Input: part model. Units: mm. Frame: model coordinates. A direction names the side the tool comes from. Give positions to 0.01 mm unless a question says otherwise; leave off trailing zeros. Write each loop counter-clockwise with the first axis right and the second up, starting at its lowest first coordinate (ties: lowest second). Pieces come first, ordered by that corner, then holes. Notation, with made-up numbers: (68, 18.5) - (73, 18.5) arc R6 ccw to (73, 26.5) - close; hole circle Ø7 at (40.5, -39.75). An arc over 180 degrees is marked (long way). Answer as a JSON object with one key per item and string values. Group by question number.
Autodesk Inventor part; units mm, degrees
ref_plane "YZ Plane" through (0, 0, 0) normal (1, 0, 0) x (0, 1, 0)
ref_plane "XZ Plane" through (0, 0, 0) normal (0, 1, 0) x (-1, 0, 0)
ref_plane "XY Plane" through (0, 0, 0) normal (0, 0, 1) x (1, 0, 0)
sketch "Boceto1" plane through (0, 0, 0) normal (0, 0, 1) x (1, 0, 0)
  line L0 (-225.8925, 111.7519) -> (-185.8925, 111.7519)
  line L1 (-185.8925, 111.7519) -> (-185.8925, 71.7519)
  line L2 (-225.8925, 101.7519) -> (-195.8925, 101.7519)
  line L3 (-195.8925, 101.7519) -> (-195.8925, 71.7519)
  line L4 (-225.8925, 101.7519) -> (-225.8925, 111.7519)
  line L5 (-195.8925, 71.7519) -> (-185.8925, 71.7519)
  point P0 (0, 0)
  point P1 (0, 4.2735)
  dimension "d1" = 10
  dimension "d3" = 10
  dimension "d4" = 30
  dimension "d7" = 40
extrude "Extrusión1" add sketch "Boceto1" along normal blind 30
properties part number "Tope_Extremos" material "Plástico ABS"
1) Pin query (flat end, axial travel): P1, Ø9, axis at x = -210.5, z = 7.5, coming from the -Y side; P2, Ø15, axis at y = 83, z = 19, coming from the -X side; P3, Ø5, axis at y = 101.5, z = 23.5, coming from the -X side; P4, Ø4, axis at x = -215, y = 98, coming from the +Z side. Return the tip coordinate at first contact, or that it passes through.
2) Cut plane A-A on z = 10.75. Return the cut outline in (x, y).
3) Cut plane C-C on x = -198. Return the cut outline in (y, z), and give its area (3 significant figures).
4) Line query: line 1 along Y through (x, z) = (-212.5, 7); line 2 along X through (y, z) = (94.5, 25.75). Output: solid intervals per line, ascending. Write a range as from..to.
5) Reachability of faces 1 (the face through (-197, 105, 0)), 2 (the face through (-195.892, 87, 15)) from +Z, -Z, +X, -X, +Y, -Y: full face, straight path, thin tool, end or side. Return the list, or none.
6) Cut plane B-B on y = 97. Return the cut outline in (x, z).
Filled in:
{
 "1": {"P1": "stops at y = 101.75", "P2": "stops at x = -195.89", "P3": "stops at x = -225.89", "P4": "passes through"},
 "2": {"outline": "(-225.89, 101.75) - (-195.89, 101.75) - (-195.89, 71.75) - (-185.89, 71.75) - (-185.89, 111.75) - (-225.89, 111.75) - close"},
 "3": {"outline": "(101.75, 0) - (111.75, 0) - (111.75, 30) - (101.75, 30) - close", "area": "300 mm²"},
 "4": {"line 1": "y = 101.75..111.75", "line 2": "x = -195.89..-185.89"},
 "5": {"face 1": "-Z, +X, -X, +Y, -Y", "face 2": "+Z, -Z, -X, -Y"},
 "6": {"outline": "(-195.89, 0) - (-185.89, 0) - (-185.89, 30) - (-195.89, 30) - close"}
}
